Read the model definition and answer for the solid it produces. Units are mm, in the model's axes. Face numbers are marked on the shaded views. Give positions to 0.01 mm unless a question says otherwise; leave off trailing zeros. Write each loop counter-clockwise with the first axis right and the second up, starting at its lowest first coordinate (ties: lowest second). Pieces come first, ordered by that corner, then holes. Notation, with made-up numbers: (53.5, -26.5) -> (101.5, -26.5) arc R6 ccw to (101.5, -16.5) -> close; hole circle Ø6 at (4, 11.25). An arc over 180 degrees is marked (long way). Answer as CSV lines item,"result". Start each with the question number.
1. Given pin 1 (2.5 mm diameter, centred on x = 133, y = -3, fed in from +Z); pin 2 (4 mm diameter, centred on x = 32, y = -5, fed in from -Z); pin 3 (1.5 mm diameter, centred on y = 17.5, z = 1.5, fed in from +X); pin 4 (1.2 mm diameter, centred on y = 1, z = -3, fed in from +X), each flat-ended and moving along its own axis, determine where each tip first touches the part or whether it passes through.
2. For a pull along X with two mould halves and no side action, classify the marked faces 1 and 2 as pulls with the +X half, pulls with the -X half, needs draft (parallel to the pull), parting line crosses it, or undercut.
3. The part is cut by section C-C, the plane x = 107.5. Determine the outline of the cut face in (y, z).
4. Find the intervals of material crossed by line 1 (Z direction, x = 125.5, y = 12); line 2 (Y direction, x = 32, z = -1.3); line 3 (Y direction, x = 32, z = -3.2), in increasing order.
5. The part is cut by section B-B, the plane z = -2.75. Determine the outline of the cut face in (x, y), and give its area (3 significant figures).
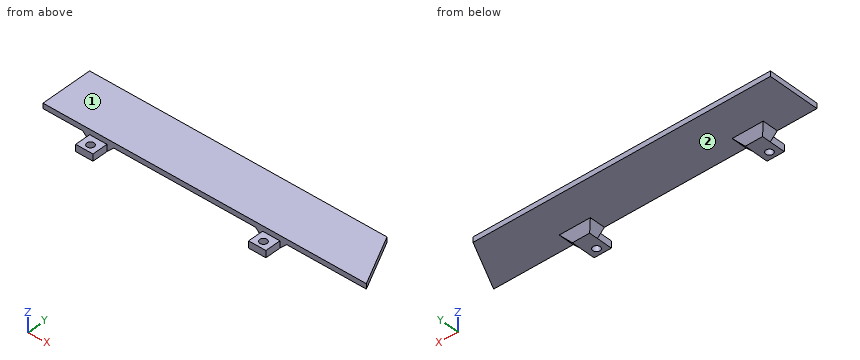
from build123d import *

# Parameters (mm, degrees)
DODANIE_WYCI_GNI_CIE1_DEPTH = 3
SZKIC2_W                    = 10
SZKIC2_H                    = 14
SZKIC2_R                    = 2.1
DODANIE_WYCI_GNI_CIE2_DEPTH = 4
SFAZOWANIE1_SIZE            = 4


with BuildPart() as part:
    # Szkic1 → Dodanie-wyciągnięcie1 (new body)
    with BuildSketch(Plane.XY):
        Polygon((0, 0), (187, 0), (171.996760863, 30), (0, 30), align=None)
    extrude(amount=DODANIE_WYCI_GNI_CIE1_DEPTH)

    # Szkic2 → Dodanie-wyciągnięcie2 (add)
    # profile 1 of 2: a face of its own
    with BuildSketch(Plane(origin=(0, 0, 0), x_dir=(-1, 0, 0), z_dir=(0, 0, -1))):
        with Locations((-132, -2)):
            Rectangle(SZKIC2_W, SZKIC2_H)
        with Locations((-132, -5)):
            Circle(SZKIC2_R, mode=Mode.SUBTRACT)
    # profile 2 of 2: a face of its own
    with BuildSketch(Plane(origin=(0, 0, 0), x_dir=(-1, 0, 0), z_dir=(0, 0, -1))):
        with Locations((-32, -2)):
            Rectangle(SZKIC2_W, SZKIC2_H)
        with Locations((-32, -5)):
            Circle(SZKIC2_R, mode=Mode.SUBTRACT)
    extrude(amount=DODANIE_WYCI_GNI_CIE2_DEPTH)

    # Sfazowanie1
    sfazowanie1_edges = [part.edges().sort_by_distance(p)[0] for p in [
        (37, 2.5, 0),
        (32, 5, 0),
        (27, 2.5, 0),
        (127, 2.5, 0),
        (132, 5, 0),
        (137, 2.5, 0),
    ]]
    chamfer(sfazowanie1_edges, length=SFAZOWANIE1_SIZE - 0.0001)  # a hair under: the kernel refuses the full size


solid = part.part
Results found:
1,pin 1,"stops at z = 0"
1,pin 2,"passes through"
1,pin 3,"stops at x = 178.62"
1,pin 4,"stops at x = 138.6"
2,face 1,"needs draft"
2,face 2,"undercut"
3,outline,"(0, 0) -> (30, 0) -> (30, 3) -> (0, 3) -> close"
4,line 1,"z = 0 to 3"
4,line 2,"y = -9 to -7.1, -2.9 to 7.7"
4,line 3,"y = -9 to -7.1, -2.9 to 5.8"
5,outline,"(25.75, 0) -> (27, 0) -> (27, -9) -> (37, -9) -> (37, 0) -> (38.25, 0) -> (38.25, 6.25) -> (25.75, 6.25) -> close; (125.75, 0) -> (127, 0) -> (127, -9) -> (137, -9) -> (137, 0) -> (138.25, 0) -> (138.25, 6.25) -> (125.75, 6.25) -> close; hole circle Ø4.2 at (32, -5); hole circle Ø4.2 at (132, -5)"
5,area,"309 mm²"
